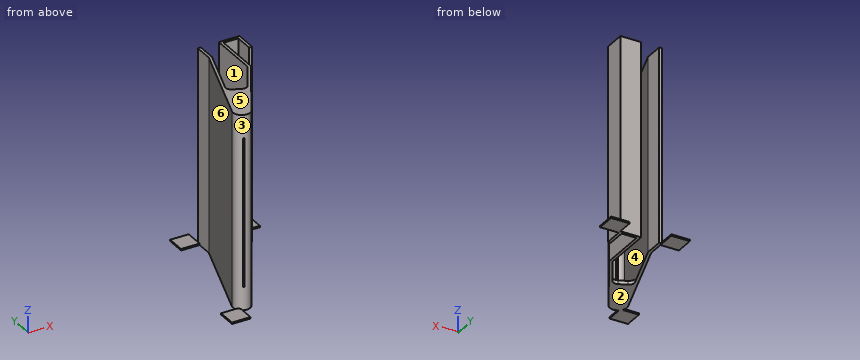
from build123d import *

# Parameters (mm, degrees)
BOSS_EXTRUDE1_DEPTH     = 105
BOSS_EXTRUDE2_DEPTH     = 2
FILLET1_R               = 3
CUT_EXTRUDE1_DEPTH      = 40
CUT_EXTRUDE1_DEPTH_BACK = 40
SKETCH4_W               = 10
SKETCH4_H               = 10
BOSS_EXTRUDE3_DEPTH     = 0.8


with BuildPart() as part:
    # Sketch1 → Boss-Extrude1 (new body)
    with BuildSketch(Plane.XY):
        with BuildLine():
            Line((0, 0), (0, 10))
            Line((0, 10), (-8, 10))
            Line((-8, 10), (-8, -15))
            Line((-8, -15), (-28.512191548, -50.528157935))
            ThreePointArc((-28.512191548, -50.528157935), (-34.418441215, -52.438299786), (-36.919980235, -46.757214542))
            Line((-36.919980235, -46.757214542), (-20.915152124, 1.6))
            Line((-20.915152124, 1.6), (-20.915152124, 11.6))
            Line((-20.915152124, 11.6), (-19.315152124, 11.6))
            Line((-19.315152124, 11.6), (-19.315152124, 1.342102465))
            Line((-19.315152124, 1.342102465), (-35.401013831, -47.259948135))
            ThreePointArc((-35.401013831, -47.259948135), (-33.763672062, -50.978410285), (-29.897832194, -49.728157935))
            Line((-29.897832194, -49.728157935), (-9.6, -14.571281292))
            Line((-9.6, -14.571281292), (-9.6, 11.6))
            Line((-9.6, 11.6), (1.6, 11.6))
            Line((1.6, 11.6), (1.6, 0))
            Line((1.6, 0), (0, 0))
        make_face()
    extrude(amount=BOSS_EXTRUDE1_DEPTH)

    # Sketch2 → Boss-Extrude2 (add)
    with BuildSketch(Plane(origin=(0, 0, 0), x_dir=(-1, 0, 0), z_dir=(0, 0, -1))):
        with BuildLine():
            Line((35.401013831, -47.259948135), (29.116843924, -28.272868091))
            Line((29.116843924, -28.272868091), (19.897832194, -32.407649859))
            Line((19.897832194, -32.407649859), (29.897832194, -49.728157935))
            ThreePointArc((29.897832194, -49.728157935), (33.763672062, -50.978410285), (35.401013831, -47.259948135))
        make_face()
    boss_extrude2 = extrude(amount=-BOSS_EXTRUDE2_DEPTH)

    # Mirror1: Boss-Extrude2 across plane
    add(boss_extrude2.mirror(Plane.XY.offset(52.5)))

    # Fillet1
    fillet1_edges = [part.edges().sort_by_distance(p)[0] for p in [
        (-19.897832194, -32.407649859, 1),
        (-29.116843924, -28.272868091, 1),
        (-29.116843924, -28.272868091, 104),
        (-19.897832194, -32.407649859, 104),
    ]]
    fillet(fillet1_edges, radius=FILLET1_R)

    # Sketch3 → Cut-Extrude1 (cut, two sides: drawn at the far end of the back side and taken through both)
    with BuildSketch(Plane.XY.offset(52.5).offset(-CUT_EXTRUDE1_DEPTH_BACK)):
        with BuildLine():
            Line((-32.143379325, -48.338130177), (-33.714421802, -53.084900187))
            ThreePointArc((-33.714421802, -53.084900187), (-34.219846801, -53.33895839), (-34.473905004, -52.833533391))
            Line((-34.473905004, -52.833533391), (-32.902862527, -48.08676338))
            ThreePointArc((-32.902862527, -48.08676338), (-32.397437528, -47.832705178), (-32.143379325, -48.338130177))
        make_face()
    extrude(amount=CUT_EXTRUDE1_DEPTH + CUT_EXTRUDE1_DEPTH_BACK, mode=Mode.SUBTRACT)

    # Sketch4 → Boss-Extrude3 (add)
    with BuildSketch(Plane(origin=(0, 0, 0), x_dir=(-1, 0, 0), z_dir=(0, 0, -1))):
        with Locations((-6.6, 15)):
            Rectangle(SKETCH4_W, SKETCH4_H)
        with Locations((25.915152124, 15)):
            Rectangle(SKETCH4_W, SKETCH4_H)
        with Locations((40.183119354, -55.872445207)):
            Rectangle(SKETCH4_W, SKETCH4_H)
    extrude(amount=-BOSS_EXTRUDE3_DEPTH)


solid = part.part
For this review, take the finished solid that the model builds, in its own axes (mm). Face numbers are marked on the shaded views. A direction names the side the tool comes from. Round coordinates to 2 decimals unless told otherwise and drop trailing zeros. Write each loop counter-clockwise with the first axis right and the second up, starting at its lowest first coordinate (ties: lowest second). Pieces come first, ordered by that corner, then holes. Notation, with made-up numbers: (15.25, 48) -> (49.25, 48) arc R28 ccw to (49.25, 68) -> close; hole circle Ø8 at (50.5, -14.75). An arc over 180 degrees is marked (long way). Use CSV: the item, a comma, the result in double quotes.
(1) To check wall thickness, follow L1, parallel to Z at x = -30, y = -34.5; L2, parallel to Y at x = 0.5, z = 51.5; L3, parallel to X at y = 0.5, z = 22. State the ranges of each line that lie inside material, in increasing order. Write a range as [from, to].
Computed values:
L1,"[0, 2], [103, 105]"
L2,"[0, 11.6]"
L3,"[-21.28, -19.59], [-9.6, -8], [0, 1.6]"
(2) Draft analysis for pull direction X (two halves, no side actions). For the marked faces 4, 5 and 6, state which applies: +X half, -X half, draft (parallel to the pull), parting line (faces both ways), or undercut.
Computed values:
face 4,"undercut"
face 5,"draft"
face 6,"-X half"
(3) Consider section B-B, the plane y = 8. Give the boundary of the cut face in (x, z).
Computed values:
outline,"(-20.92, 0) -> (-19.32, 0) -> (-19.32, 105) -> (-20.92, 105) -> close; (-9.6, 0) -> (-8, 0) -> (-8, 105) -> (-9.6, 105) -> close; (0, 0) -> (1.6, 0) -> (1.6, 105) -> (0, 105) -> close"
(4) For the marked faces 1, 2 and 3, list the 3-axis set-ups (+Z, -Z, +X, -X, +Y, -Y) from which the entire face can be reached by the end or side of a thin tool; tool diameter is ignored.
Computed values:
face 1,"+Z, -Z, +Y"
face 2,"-Z, +X, -X, +Y, -Y"
face 3,"+Z"
(5) Clearance check with flat-ended pins moving along their axes: P1, Ø5, axis at y = -44, z = 46, coming from the +X side; P2, Ø9, axis at x = -5, z = 49.5, coming from the -Y side; P3, Ø5, axis at y = 5.5, z = 45, coming from the -X side. State where each tip first meets the part, or that it passes through.
Computed values:
P1,"x = -23.3"
P2,"y = -17.6"
P3,"x = -20.92"
(6) Consider section D-D, the plane x = 5. Give the boundary of the cut face in (y, z).
Computed values:
outline,"(10, 0) -> (20, 0) -> (20, 0.8) -> (10, 0.8) -> close"
(7) Consider section C-C, the plane y = -6.5. Give the boundary of the cut face in (x, z), plus the area to 3 significant figures.
Computed values:
outline,"(-23.6, 0) -> (-21.91, 0) -> (-21.91, 105) -> (-23.6, 105) -> close; (-9.6, 0) -> (-8, 0) -> (-8, 105) -> (-9.6, 105) -> close"
area,"345 mm²"
(8) Consider section A-A, the plane z = 27.5. Give the boundary of the cut face in (x, y), plus the area to 3 significant figures.
Computed values:
outline,"(-36.92, -46.76) arc R4.63 ccw to (-34.35, -52.47) -> (-33.85, -50.94) arc R3.03 cw to (-35.4, -47.26) -> (-19.32, 1.34) -> (-19.32, 11.6) -> (-20.92, 11.6) -> (-20.92, 1.6) -> close; (-33.59, -52.72) arc R4.63 ccw to (-28.51, -50.53) -> (-8, -15) -> (-8, 10) -> (0, 10) -> (0, 0) -> (1.6, 0) -> (1.6, 11.6) -> (-9.6, 11.6) -> (-9.6, -14.57) -> (-29.9, -49.73) arc R3.03 cw to (-33.09, -51.19) -> close"
area,"254 mm²"
